Source: CAD feature listing. Evaluate the final solid. Frame: model axes, mm. A direction names the side the tool comes from. Give positions to 0.01 mm unless a question says otherwise; leave off trailing zeros. Order: outer loops, then holes, each group sorted by start corner. A loop starts at its lowest first (then second) coordinate and runs counter-clockwise, first axis right, second up. Notation, with made-up numbers: (17.5, -6) - (53.5, -6) arc R30 cw to (53.5, 27) - close; hole circle Ø2 at (-15.75, 85.25). An arc over 180 degrees is marked (long way). Write each question's results on one line, items separated by ' | '. Start each with the question number.
Item 1: Contact query for flat-ended pins moving along their axis: pin 1 Ø12 at (x, z) = (33.5, -19) entering from -Y; pin 2 Ø4.5 at (x, y) = (26.8, 9.62) entering from +Z (3 decimals); pin 3 Ø4 at (x, y) = (30.8, -7.12) entering from +Z; pin 4 Ø2 at (x, z) = (7.5, -30) entering from +Y. Output: stop coordinate, or through.
Item 2: Mould query, pull axis X, two halves, no side actions, for faces 4 (the flat face through (19, 21, 0)), 5 (the flat face through (38.1, 2, -26)), 6 (the flat face through (0, 2, -26)), 7 (the conical face through (30.09, -9.38, -52.35)). Classes: released by +X, released by -X, zero draft, split by the parting line, or undercut.
Item 3: Section B-B on z = -4.5. Output: boundary loops of the cut face in (x, y).
Item 4: Line query: line 1 along Z through (x, y) = (36.5, -3) (3 decimals); line 2 along Y through (x, z) = (3.5, -23); line 3 along Y through (x, z) = (11.3, 2.1). Output: solid intervals per line, ascending.
Item 5: Set-up query: faces 1 (the flat face through (19, 3.994, -27)), 2 (the flat face through (19, 0.819, -24)), 3 (the flat face through (19, -11.881, -52)). Return all of +Z, -Z, +X, -X, +Y, -Y with unobstructed straight access to the full face (end or side cutting, diameter ignored); none if empty.
Item 6: Section A-A on x = 21.5. Output: boundary loops of the cut face in (y, z) (3 decimals).
Item 7: Section C-C on y = 19.5. Output: boundary loops of the cut face in (x, z) (3 decimals), and give its area (3 significant figures).
```python
from build123d import *

# Parameters (mm, degrees)
BOSS_EXTRUDE1_DEPTH                       = 38.1
CSK_FOR_8_FLAT_HEAD_MACHINE_SCREW_2_COUNT = 2
CSK_FOR_8_FLAT_HEAD_MACHINE_SCREW_2_PITCH = 23.495
CUT_EXTRUDE1_START                        = -3.175
CUT_EXTRUDE1_OUTLINE_R                    = 6.35
CUT_EXTRUDE1_DEPTH                        = 3.175
M3_CLEARANCE_HOLE1_D                      = 3.4


# Read off the part's stored shape, not the designer's step: Cut-Extrude1
with BuildPart() as part:
    # Sketch1 → Boss-Extrude1 (new body)
    with BuildSketch(Plane(origin=(0, 0, 0), x_dir=(0, 0, -1), z_dir=(1, 0, 0))):
        with BuildLine():
            Line((0, 42.094372261), (0, 6.675328802))
            ThreePointArc((0, 6.675328802), (0.785233991, 4.779606252), (2.680956542, 3.994372261))
            Line((2.680956542, 3.994372261), (51.435, 3.994372261))
            ThreePointArc((51.435, 3.994372261), (53.231051224, 3.250423485), (53.975, 1.454372261))
            Line((53.975, 1.454372261), (53.975, -11.880627739))
            Line((53.975, -11.880627739), (50.8, -11.880627739))
            Line((50.8, -11.880627739), (50.8, -1.720627739))
            ThreePointArc((50.8, -1.720627739), (50.056051224, 0.075423485), (48.26, 0.819372261))
            Line((48.26, 0.819372261), (-0.494043458, 0.819372261))
            ThreePointArc((-0.494043458, 0.819372261), (-2.389766009, 1.604606252), (-3.175, 3.500328802))
            Line((-3.175, 3.500328802), (-3.175, 42.094372261))
            Line((-3.175, 42.094372261), (0, 42.094372261))
        make_face()
    extrude(amount=BOSS_EXTRUDE1_DEPTH)

    # Sketch10 → CSK for _8 Flat Head Machine Screw _100 (revolve, cut)
    with BuildSketch(Plane(origin=(7.3025, -7.118127739, -50.8), x_dir=(0, -1, 0), z_dir=(1, 0, 0))):
        Polygon((0, 0), (0, 3.175), (2.2479, 3.175), (2.2479, 1.651767624), (4.2164, 0), align=None)
    csk_for_8_flat_head_machine_screw_100 = revolve(axis=Axis((7.3025, -7.118127739, -44.45), (0, 0, -1)), mode=Mode.SUBTRACT)

    # CSK for _8 Flat Head Machine Screw _ 2: CSK for _8 Flat Head Machine Screw _100 ×2
    with Locations(*[(i * CSK_FOR_8_FLAT_HEAD_MACHINE_SCREW_2_PITCH, 0, 0) for i in range(1, CSK_FOR_8_FLAT_HEAD_MACHINE_SCREW_2_COUNT)]):
        add(csk_for_8_flat_head_machine_screw_100, mode=Mode.SUBTRACT)

    # Cut-Extrude1 outline → Cut-Extrude1 (cut)
    with BuildSketch(Plane.XY.offset(3.175).offset(CUT_EXTRUDE1_START)):
        with BuildLine():
            ThreePointArc((0, 23.044372261), (5.579615818, 36.514756443), (19.05, 42.094372261))
            Line((19.05, 42.094372261), (0, 42.094372261))
            Line((0, 42.094372261), (0, 23.044372261))
        make_face()
        with BuildLine():
            ThreePointArc((19.05, 42.094372261), (32.520384182, 36.514756443), (38.1, 23.044372261))
            Line((38.1, 23.044372261), (38.1, 42.094372261))
            Line((38.1, 42.094372261), (19.05, 42.094372261))
        make_face()
        with Locations((19.05, 30.044372261)):
            Circle(CUT_EXTRUDE1_OUTLINE_R)
    extrude(amount=CUT_EXTRUDE1_DEPTH, mode=Mode.SUBTRACT)

    # M3 Clearance Hole1 (through all)
    with Locations(Plane.XY.offset(3.175)):
        with Locations((3.55, 23.044372261), (34.55, 23.044372261), (26.8, 9.620978502), (11.3, 9.620978502)):
            Hole(M3_CLEARANCE_HOLE1_D / 2)


solid = part.part
```
Evaluation:
1) pin 1: stops at y = 0.82 | pin 2: stops at z = 3.175 | pin 3: passes through | pin 4: stops at y = 3.99
2) face 4: zero draft | face 5: released by +X | face 6: released by -X | face 7: undercut
3) outline: (0, 0.82) - (38.1, 0.82) - (38.1, 3.99) - (0, 3.99) - close
4) line 1: z = -53.975 to -50.8 | line 2: y = 0.82 to 3.99 | line 3: y = 1.35 to 7.92, 11.32 to 40.45
5) face 1: -Z, +X, -X, +Y | face 2: +Z, +X, -X, -Y | face 3: +Z, -Z, +X, -X, -Y
6) outline: (-11.881, -53.975) - (1.454, -53.975) arc R2.54 ccw to (3.994, -51.435) - (3.994, -2.681) arc R2.681 cw to (6.675, 0) - (24.186, 0) - (24.186, 3.175) - (3.5, 3.175) arc R2.681 ccw to (0.819, 0.494) - (0.819, -48.26) arc R2.54 cw to (-1.721, -50.8) - (-11.881, -50.8) - close; (35.903, 0) - (41.936, 0) - (41.936, 3.175) - (35.903, 3.175) - close
7) outline: (0, 0) - (38.1, 0) - (38.1, 3.175) - (0, 3.175) - close | area: 121 mm^2
